```python
from build123d import *

# Parameters (mm, degrees)
STOCK_PAYLOAD_BAY_1_START = 299.99
STOCK_PAYLOAD_BAY_1_DEPTH = 300.010025
CUT_EXTRUDE2_DEPTH        = 30
SKETCH1_W                 = 185.207649842
SKETCH1_H                 = 240.010025
CUT_EXTRUDE1_DEPTH        = 30


# Read off the part's stored shape, not the designer's step: Stock-Payload_bay-1
with BuildPart() as part:
    # Stock-Payload_bay-1 outline → Stock-Payload_bay-1 (new body)
    with BuildSketch(Plane.XY.offset(STOCK_PAYLOAD_BAY_1_START)):
        with BuildLine():
            Line((94.203991807, 98.4), (94.203991807, 100))
            Line((94.203991807, 100), (-94.203991807, 100))
            Line((-94.203991807, 100), (-94.203991807, 98.4))
            ThreePointArc((-94.203991807, 98.4), (-94.43235321, 97.251949701), (-95.082671465, 96.278679653))
            Line((-95.082671465, 96.278679653), (-111.640030762, 79.721320356))
            ThreePointArc((-111.640030762, 79.721320356), (-112.290349017, 76.45194971), (-109.518710415, 74.600000005))
            Line((-109.518710415, 74.600000005), (-97.203991812, 74.600000005))
            ThreePointArc((-97.203991812, 74.600000005), (-95.082671465, 73.721320347), (-94.203991807, 71.6))
            Line((-94.203991807, 71.6), (-94.203991807, 70))
            ThreePointArc((-94.203991807, 70), (-93.735146897, 68.868608907), (-92.603658035, 68.4))
            Line((-92.603658035, 68.4), (92.603991807, 68.4))
            ThreePointArc((92.603991807, 68.4), (93.735362657, 68.86862915), (94.203991807, 70))
            Line((94.203991807, 70), (94.203991807, 71.6))
            ThreePointArc((94.203991807, 71.6), (95.082671465, 73.721320347), (97.203991812, 74.600000005))
            Line((97.203991812, 74.600000005), (109.518710415, 74.600000005))
            ThreePointArc((109.518710415, 74.600000005), (112.290349017, 76.45194971), (111.640030762, 79.721320356))
            Line((111.640030762, 79.721320356), (95.082671465, 96.278679653))
            ThreePointArc((95.082671465, 96.278679653), (94.43235321, 97.251949701), (94.203991807, 98.4))
        make_face()
    extrude(amount=STOCK_PAYLOAD_BAY_1_DEPTH)

    # Sketch2 → Cut-Extrude2 (cut)
    with BuildSketch(Plane(origin=(0, 100, 0), x_dir=(1, 0, 0), z_dir=(0, 1, 0))):
        with BuildLine():
            Line((-50, -306.99), (50, -306.99))
            ThreePointArc((50, -306.99), (60, -316.99), (50, -326.99))
            Line((50, -326.99), (-50, -326.99))
            ThreePointArc((-50, -326.99), (-60, -316.99), (-50, -306.99))
        make_face()
        with BuildLine():
            Line((-50, -593.000025), (50, -593.000025))
            ThreePointArc((50, -593.000025), (60, -583.000025), (50, -573.000025))
            Line((50, -573.000025), (-50, -573.000025))
            ThreePointArc((-50, -573.000025), (-60, -583.000025), (-50, -593.000025))
        make_face()
    extrude(amount=-CUT_EXTRUDE2_DEPTH, mode=Mode.SUBTRACT)

    # Sketch1 → Cut-Extrude1 (cut)
    with BuildSketch(Plane(origin=(0, 68.4, 0), x_dir=(-1, 0, 0), z_dir=(0, -1, 0))):
        with Locations((-0.000166886, -449.9950125)):
            Rectangle(SKETCH1_W, SKETCH1_H)
    extrude(amount=-CUT_EXTRUDE1_DEPTH, mode=Mode.SUBTRACT)


solid = part.part
```
Check sheet for the modelled part. Datum: model origin and axes. Units: mm. A direction names the side the tool comes from. Coordinates: 2 decimals unless noted, no trailing zeros. Order: outer loops, then holes, each group sorted by start corner. A loop starts at its lowest first (then second) coordinate and runs counter-clockwise, first axis right, second up. Notation, with made-up numbers: M 71.5,4 L 85.5,4 A36 cw 85.5,39 Z; hole C 19,50 d8. An arc over 180 degrees is marked long. One line per question, with ' | ' between items. Start each with the question number.
Item 1: Gauge pin test, flat ends, axial feed: P1, Ø1.5, axis at y = 80, z = 525.5, coming from the -X side; P2, Ø15, axis at y = 85.5, z = 501.5, coming from the -X side; P3, Ø1, axis at y = 92.5, z = 443, coming from the +X side. Record the tip position at first contact, or that the pin passes through.
Item 2: Sectioned sample at A-A on z = 423.5. Record the cut outline in (x, y).
Item 3: Sectioned sample at C-C on y = 91. Record the cut outline in (x, z).
Item 4: Material ranges on line 1 (Z direction, x = 35.5, y = 75); line 2 (Z direction, x = -80, y = 87); line 3 (X direction, y = 98, z = 423), recorded low to high.
Item 5: Sectioned sample at B-B on x = 70.5. Record the cut outline in (y, z), and give its area (3 significant figures).
Item 6: Access from +Z, -Z, +X, -X, +Y, -Y to the whole of each face (thin tool, end or side, straight path). Record for faces 4 (the flat face through (-1, 85, 306.99)), 5 (the flat face through (1, 83, 329.99)), 6 (the flat face through (-103, 74.6, 448)), 7 (the flat face through (103, 74.6, 448)).
Item 7: Sectioned sample at D-D on x = -10.5. Record the cut outline in (y, z).
Item 8: Mould release check, pull along Z, two halves, no side actions. Record for faces 1 (the flat face through (-2, 84, 299.99)), 2 (the flat face through (1, 83, 570)), 3 (the flat face through (103.48, 87.88, 447.89)): pulls with the +Z half, pulls with the -Z half, needs draft (parallel to the pull), parting line crosses it, or undercut.
Answer below:
1) P1: stops at x = -112.02 | P2: stops at x = -112.49 | P3: stops at x = 99.36
2) outline: M -111.64,79.72 A3 ccw -109.52,74.6 L -97.2,74.6 A3 cw -94.2,71.6 L -94.2,70 A1.6 ccw -92.6,68.4 L -92.6,98.4 L 92.6,98.4 L 92.6,68.4 A1.6 ccw 94.2,70 L 94.2,71.6 A3 cw 97.2,74.6 L 109.52,74.6 A3 ccw 111.64,79.72 L 95.08,96.28 A3 cw 94.2,98.4 L 94.2,100 L -94.2,100 L -94.2,98.4 A3 cw -95.08,96.28 Z
3) outline: M -100.36,299.99 L 100.36,299.99 L 100.36,600 L -100.36,600 Z; hole M -92.6,329.99 L 92.6,329.99 L 92.6,570 L -92.6,570 Z; hole M -50,306.99 L 50,306.99 A10 ccw 50,326.99 L -50,326.99 A10 ccw Z; hole M -50,573 L 50,573 A10 ccw 50,593 L -50,593 A10 ccw Z
4) line 1: z = 299.99 to 306.99, 326.99 to 329.99, 570 to 573, 593 to 600 | line 2: z = 299.99 to 329.99, 570 to 600 | line 3: x = -94.23 to -92.6, 92.6 to 94.23
5) outline: M 68.4,299.99 L 100,299.99 L 100,600 L 68.4,600 L 68.4,570 L 98.4,570 L 98.4,329.99 L 68.4,329.99 Z | area: 2,280 mm^2
6) face 4: +Y | face 5: -Y | face 6: +Z, -Z, -X, -Y | face 7: +Z, -Z, +X, -Y
7) outline: M 68.4,299.99 L 100,299.99 L 100,306.99 L 70,306.99 L 70,326.99 L 100,326.99 L 100,573 L 70,573 L 70,593 L 100,593 L 100,600 L 68.4,600 L 68.4,570 L 98.4,570 L 98.4,329.99 L 68.4,329.99 Z
8) face 1: pulls with the -Z half | face 2: undercut | face 3: needs draft
